Input: part model. Units: mm. Frame: model coordinates. A direction names the side the tool comes from. Round coordinates to 2 decimals unless told otherwise and drop trailing zeros. Loops run counter-clockwise (first coordinate to the right, second up) from the corner with the lowest first, then second, coordinate; pieces in that order, holes last.
(1) Line query: line 1 (X direction, y = 16.5, z = 33) (3 decimals); line 2 (Y direction, x = 51.5, z = 21); line 3 (Y direction, x = -5, z = 22). Output: solid intervals per line, ascending.
(2) Cut plane B-B, the plane z = 34. Output: boundary loops of the cut face in (x, y) (3 decimals), and give its area (3 significant figures).
(3) First-contact query: pin 1 Ø22 at (y, z) = (10.5, 22.5) entering from +X (3 decimals); pin 2 Ø22 at (x, z) = (-70.5, 22) entering from -Y; pin 3 Ø4 at (y, z) = (16.5, 11.5) entering from -X (3 decimals). Flat tips, straight axial feed; report the tip coordinate or a pass-through.
(4) Cut plane C-C, the plane x = -13.5. Output: boundary loops of the cut face in (y, z), and give its area (3 significant figures).
(5) Cut plane A-A, the plane y = 14. Output: boundary loops of the cut face in (x, z) (3 decimals).
(6) Access query for faces 1 (the face through (-22.225, 29, 22)), 2 (the face through (-28.575, 22, 22)), 3 (the face through (61, 51.587, 22)). Directions: +Z, -Z, +X, -X, +Y, -Y. A direction counts if a zero-diameter tool reaches every point of the face in a straight line with its end or side. Return the directions, or none.
(7) Cut plane D-D, the plane x = -43.5. Output: boundary loops of the cut face in (y, z), and give its area (3 significant figures).
(8) Draft query along Z for faces 4 (the face through (28, 33, 0)), 5 (the face through (-86.31, 54.72, 19.83)), 6 (the face through (0, -6.35, 22)). Return one class per face: released by +Z, released by -Z, zero draft, split by the parting line, or undercut.
from build123d import *

# Parameters (mm, degrees)
BOSS_EXTRUDE1_DEPTH = 44.45
SKETCH2_R           = 3.937
CUT_EXTRUDE1_DEPTH  = 118.517447401


with BuildPart() as part:
    # Sketch1 → Boss-Extrude1 (new body)
    with BuildSketch(Plane.XY):
        Polygon((-22.225, 0), (22.225, 0), (22.225, 57.9374), (28.575, 57.9374), (92.075, 57.9374), (92.075, 51.5874), (28.575, 51.5874), (28.575, -6.35), (-28.575, -6.35), (-28.575, 51.5874), (-92.075, 51.5874), (-92.075, 57.9374), (-28.575, 57.9374), (-22.225, 57.9374), align=None)
    extrude(amount=BOSS_EXTRUDE1_DEPTH)

    # Sketch2 → Cut-Extrude1 (cut, through all)
    with BuildSketch(Plane.XZ.offset(-51.5874)):
        with Locations((83.185, 22.225)):
            Circle(SKETCH2_R)
        with Locations((-83.185, 22.225)):
            Circle(SKETCH2_R)
    extrude(amount=-CUT_EXTRUDE1_DEPTH, mode=Mode.SUBTRACT)


solid = part.part
Reported:
1. line 1: x = -28.575 to -22.225, 22.225 to 28.575
1. line 2: y = 51.59 to 57.94
1. line 3: y = -6.35 to 0
2. outline: (-92.075, 51.587) - (-28.575, 51.587) - (-28.575, -6.35) - (28.575, -6.35) - (28.575, 51.587) - (92.075, 51.587) - (92.075, 57.937) - (22.225, 57.937) - (22.225, 0) - (-22.225, 0) - (-22.225, 57.937) - (-92.075, 57.937) - close
2. area: 1,910 mm2
3. pin 1: stops at x = 28.575
3. pin 2: stops at y = 51.59
3. pin 3: stops at x = -28.575
4. outline: (-6.35, 0) - (0, 0) - (0, 44.45) - (-6.35, 44.45) - close
4. area: 282 mm2
5. outline: (-28.575, 0) - (-22.225, 0) - (-22.225, 44.45) - (-28.575, 44.45) - close; (22.225, 0) - (28.575, 0) - (28.575, 44.45) - (22.225, 44.45) - close
6. face 1: +Z, -Z, +Y
6. face 2: +Z, -Z, -X, -Y
6. face 3: +Z, -Z, +X, -Y
7. outline: (51.59, 0) - (57.94, 0) - (57.94, 44.45) - (51.59, 44.45) - close
7. area: 282 mm2
8. face 4: released by -Z
8. face 5: undercut
8. face 6: zero draft
